from build123d import *

# Parameters (mm, degrees)
SKETCH002_W     = 64.5
SKETCH002_H     = 43
PAD001_DEPTH    = 25
THICKNESS_T     = -1
FILLET001_R     = 5
SKETCH008_W     = 43
SKETCH008_H     = 25
PAD006_DEPTH    = 22
SKETCH009_W     = 18
SKETCH009_H     = 39
POCKET002_DEPTH = 10
FILLET005_R     = 3
FILLET006_R     = 2


with BuildPart() as part:
    # Sketch002 → Pad001 (new body)
    with BuildSketch(Plane.XY):
        Rectangle(SKETCH002_W, SKETCH002_H)
    extrude(amount=PAD001_DEPTH)

    # Thickness
    thickness_openings = [part.faces().sort_by_distance(p)[0] for p in [
        (0, 0, 25),
    ]]
    offset(amount=THICKNESS_T, openings=thickness_openings)

    # Fillet001
    fillet001_edges = [part.edges().sort_by_distance(p)[0] for p in [
        (0, 20.5, 1),
        (31.25, 0, 1),
        (0, -20.5, 1),
        (-31.25, 0, 1),
    ]]
    fillet(fillet001_edges, radius=FILLET001_R)

    # Sketch008 (on DatumPlane) → Pad006 (join)
    with BuildSketch(Plane.YZ.offset(32.25)):
        with Locations((0, 12.5)):
            Rectangle(SKETCH008_W, SKETCH008_H)
    extrude(amount=PAD006_DEPTH)

    # Sketch009 (on DatumPlane) → Pocket002 (cut)
    with BuildSketch(Plane.XY.offset(25)):
        with Locations((43.25, 0)):
            Rectangle(SKETCH009_W, SKETCH009_H)
    extrude(amount=-POCKET002_DEPTH, mode=Mode.SUBTRACT)

    # Fillet005
    fillet005_edges = [part.edges().sort_by_distance(p)[0] for p in [
        (43.25, 19.5, 15),
        (52.25, 0, 15),
        (43.25, -19.5, 15),
        (34.25, 0, 15),
    ]]
    fillet(fillet005_edges, radius=FILLET005_R)

    # Fillet006
    fillet006_edges = [part.edges().sort_by_distance(p)[0] for p in [
        (0, 21.5, 0),
        (32.25, 0, 0),
        (0, -21.5, 0),
        (-32.25, 0, 0),
        (43.25, 21.5, 0),
        (43.25, -21.5, 0),
        (54.25, 0, 0),
    ]]
    fillet(fillet006_edges, radius=FILLET006_R)


solid = part.part
Model file for the job. Use its own axes, mm. A direction names the side the tool comes from. Round coordinates to 2 decimals unless told otherwise and drop trailing zeros. Order: outer loops, then holes, each group sorted by start corner. A loop starts at its lowest first (then second) coordinate and runs counter-clockwise, first axis right, second up.
(1) Pin check, flat tip, straight feed: pin 1 (9.5 mm diameter, centred on x = 42, y = 2, fed in from +Z). Stop position of the tip, or through.
(2) 3-axis set-ups, long thin cutter, end or side, ignore diameter. For faces 1 (the face through (51.39, 0.27, 15.9)), 2 (the face through (33, 0, 25)): which of +Z, -Z, +X, -X, +Y, -Y reach the whole face in a straight line?
(3) Band-saw the part on C-C (y = 2). List the corners of the cut face in (x, z).
(4) Band-saw the part on A-A (z = 7). List the corners of the cut face in (x, y).
(5) Pull direction Y, two halves, no side cores. Call faces 3 (the face through (-31.25, 0, 15)), 4 (the face through (10, -21.5, 13)), 5 (the face through (-31.68, 0.3, 0.6)), 6 (the face through (11.61, 20.93, 0.6)): released by +Y, released by -Y, zero draft, split by the parting line, or undercut.
(6) Band-saw the part on D-D (z = 19.5). List the corners of the cut face in (x, y), then the cut area to 3 significant figures.
(7) Drill centre lines: line 1 (X direction, y = 13, z = 24); line 2 (X direction, y = -4, z = 14.5); line 3 (Y direction, x = -7.5, z = 17.5). Where is each one in solid material? Low to high.
(8) Band-saw the part on B-B (x = 45). List the corners of the cut face in (y, z), then the cut area to 3 significant figures.
Verdict:
1. pin 1: stops at z = 15
2. face 1: +Z
2. face 2: +Z, +X, -X, +Y, -Y
3. outline: (-32.25, 2) arc R2 ccw to (-30.25, 0) - (52.25, 0) arc R2 ccw to (54.25, 2) - (54.25, 25) - (52.25, 25) - (52.25, 18) arc R3 cw to (49.25, 15) - (37.25, 15) arc R3 cw to (34.25, 18) - (34.25, 25) - (31.25, 25) - (31.25, 6) arc R5 cw to (26.25, 1) - (-26.25, 1) arc R5 cw to (-31.25, 6) - (-31.25, 25) - (-32.25, 25) - close
4. outline: (-32.25, -21.5) - (54.25, -21.5) - (54.25, 21.5) - (-32.25, 21.5) - close; hole (-31.25, -20.5) - (31.25, -20.5) - (31.25, 20.5) - (-31.25, 20.5) - close
5. face 3: undercut
5. face 4: released by -Y
5. face 5: zero draft
5. face 6: released by +Y
6. outline: (-32.25, -21.5) - (54.25, -21.5) - (54.25, 21.5) - (-32.25, 21.5) - close; hole (-31.25, -20.5) - (31.25, -20.5) - (31.25, 20.5) - (-31.25, 20.5) - close; hole (34.25, -19.5) - (52.25, -19.5) - (52.25, 19.5) - (34.25, 19.5) - close
6. area: 455 mm2
7. line 1: x = -32.25 to -31.25, 31.25 to 34.25, 52.25 to 54.25
7. line 2: x = -32.25 to -31.25, 31.25 to 54.25
7. line 3: y = -21.5 to -20.5, 20.5 to 21.5
8. outline: (-21.5, 2) arc R2 ccw to (-19.5, 0) - (19.5, 0) arc R2 ccw to (21.5, 2) - (21.5, 25) - (19.5, 25) - (19.5, 18) arc R3 cw to (16.5, 15) - (-16.5, 15) arc R3 cw to (-19.5, 18) - (-19.5, 25) - (-21.5, 25) - close
8. area: 687 mm2
